Build history of the part. All positions in model axes, mm. Face numbers are marked on the shaded views. A direction names the side the tool comes from. Give positions to 0.01 mm unless a question says otherwise; leave off trailing zeros. Use a Markdown table: item, result.
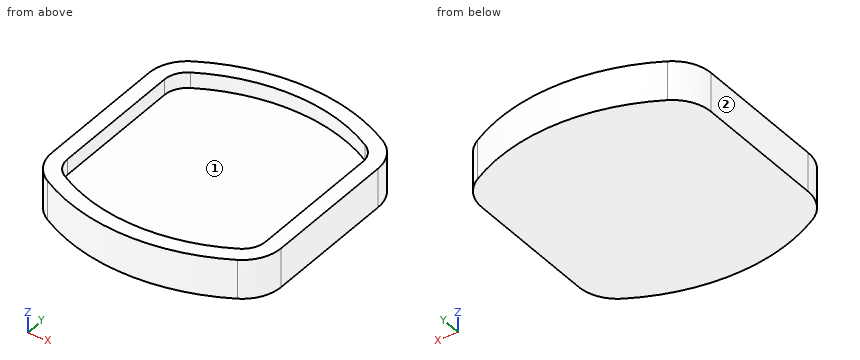
from build123d import *

# Parameters (mm, degrees)
F1_DEPTH = 6.35
F3_DEPTH = 9.525


with BuildPart() as f1:
    # F0 (on Top) → F1 (new body)
    with BuildSketch(Plane.XY):
        with BuildLine():
            Line((46.6725, -27.735808), (46.6725, 27.735808))
            ThreePointArc((46.6725, 27.735808), (44.518987, 35.719317), (38.642716, 41.536831))
            ThreePointArc((38.642716, 41.536831), (0, 51.7525), (-38.642716, 41.536831))
            ThreePointArc((-38.642716, 41.536831), (-44.518987, 35.719317), (-46.6725, 27.735808))
            Line((-46.6725, 27.735808), (-46.6725, -27.735808))
            ThreePointArc((-46.6725, -27.735808), (-44.518987, -35.719317), (-38.642716, -41.536831))
            ThreePointArc((-38.642716, -41.536831), (0, -51.7525), (38.642716, -41.536831))
            ThreePointArc((38.642716, -41.536831), (44.518987, -35.719317), (46.6725, -27.735808))
        make_face()
        with BuildLine():
            ThreePointArc((-35.504629, -36.016422), (-39.030392, -32.525914), (-40.3225, -27.735808))
            Line((-40.3225, -27.735808), (-40.3225, 27.735808))
            ThreePointArc((-40.3225, 27.735808), (-39.030392, 32.525914), (-35.504629, 36.016422))
            ThreePointArc((-35.504629, 36.016422), (0, 45.4025), (35.504629, 36.016422))
            ThreePointArc((35.504629, 36.016422), (39.030392, 32.525914), (40.3225, 27.735808))
            Line((40.3225, 27.735808), (40.3225, -27.735808))
            ThreePointArc((40.3225, -27.735808), (39.030392, -32.525914), (35.504629, -36.016422))
            ThreePointArc((35.504629, -36.016422), (0, -45.4025), (-35.504629, -36.016422))
        make_face(mode=Mode.SUBTRACT)
    extrude(amount=F1_DEPTH)

    # F2 (on Top) → F3 (join)
    with BuildSketch(Plane.XY):
        with BuildLine():
            ThreePointArc((38.642716, -41.536831), (44.518987, -35.719317), (46.6725, -27.735808))
            Line((46.6725, -27.735808), (46.6725, 27.735808))
            ThreePointArc((46.6725, 27.735808), (44.518987, 35.719317), (38.642716, 41.536831))
            ThreePointArc((38.642716, 41.536831), (0, 51.7525), (-38.642716, 41.536831))
            ThreePointArc((-38.642716, 41.536831), (-44.518987, 35.719317), (-46.6725, 27.735808))
            Line((-46.6725, 27.735808), (-46.6725, -27.735808))
            ThreePointArc((-46.6725, -27.735808), (-44.518987, -35.719317), (-38.642716, -41.536831))
            ThreePointArc((-38.642716, -41.536831), (0, -51.7525), (38.642716, -41.536831))
        make_face()
    extrude(amount=-F3_DEPTH)


solid = f1.part
1) Pin check, flat tips, straight feed: P1, Ø1, axis at x = -36, y = 16.5, coming from the +Z side; P2, Ø2, axis at y = 32, z = -4, coming from the -X side; P3, Ø4, axis at x = 30.5, z = 3, coming from the -Y side. Stop position of each tip, or through.
Computed:
| item | result |
|---|---|
| P1 | stops at z = 0 |
| P2 | stops at x = -46.33 |
| P3 | stops at y = -46.37 |
2) Tool access for the marked faces 1 and 2: list every direction of +Z, -Z, +X, -X, +Y, -Y with a clear straight run to the whole face (end or side of a thin tool).
Computed:
| item | result |
|---|---|
| face 1 | +Z |
| face 2 | +Z, -Z, -X, +Y, -Y |
3) Wall check: line 1 (X direction, y = 6, z = 4.25); line 2 (Z direction, x = 36.5, y = 17) (3 decimals); line 3 (Y direction, x = 14.5, z = 3). Give the ranges that are in metal, low to high. Write a range as from..to.
Computed:
| item | result |
|---|---|
| line 1 | x = -46.67..-40.32, 40.32..46.67 |
| line 2 | z = -9.525..0 |
| line 3 | y = -50.4..-43.92, 43.92..50.4 |
